from build123d import *

# Parameters (mm, degrees)
EXTRUDE_3_DEPTH = 550


with BuildPart() as part:
    # Эскиз1 → Вытянуть-Тонкостенный3 (new body)
    with BuildSketch(Plane(origin=(0, 0, 0), x_dir=(0, 0, -1), z_dir=(1, 0, 0))):
        with BuildLine():
            Line((8, 14), (8, 16))
            ThreePointArc((8, 16), (7.707106781, 16.707106781), (7, 17))
            Line((7, 17), (-0.5, 17))
            ThreePointArc((-0.5, 17), (-1.207106781, 16.707106781), (-1.5, 16))
            Line((-1.5, 16), (-1.5, 7.5))
            ThreePointArc((-1.5, 7.5), (-1.207106781, 6.792893219), (-0.5, 6.5))
            Line((-0.5, 6.5), (0, 6.5))
            Line((0, 6.5), (0, -6.5))
            Line((0, -6.5), (-0.5, -6.5))
            ThreePointArc((-0.5, -6.5), (-1.207106781, -6.792893219), (-1.5, -7.5))
            Line((-1.5, -7.5), (-1.5, -16))
            ThreePointArc((-1.5, -16), (-1.207106781, -16.707106781), (-0.5, -17))
            Line((-0.5, -17), (7, -17))
            ThreePointArc((7, -17), (7.707106781, -16.707106781), (8, -16))
            Line((8, -16), (8, -14))
            Line((8, -14), (6.8, -14))
            Line((6.8, -14), (6.8, -15.8))
            Line((6.8, -15.8), (-0.3, -15.8))
            Line((-0.3, -15.8), (-0.3, -7.7))
            Line((-0.3, -7.7), (1.2, -7.7))
            Line((1.2, -7.7), (1.2, 7.7))
            Line((1.2, 7.7), (-0.3, 7.7))
            Line((-0.3, 7.7), (-0.3, 15.8))
            Line((-0.3, 15.8), (6.8, 15.8))
            Line((6.8, 15.8), (6.8, 14))
            Line((6.8, 14), (8, 14))
        make_face()
    extrude(amount=EXTRUDE_3_DEPTH)


solid = part.part
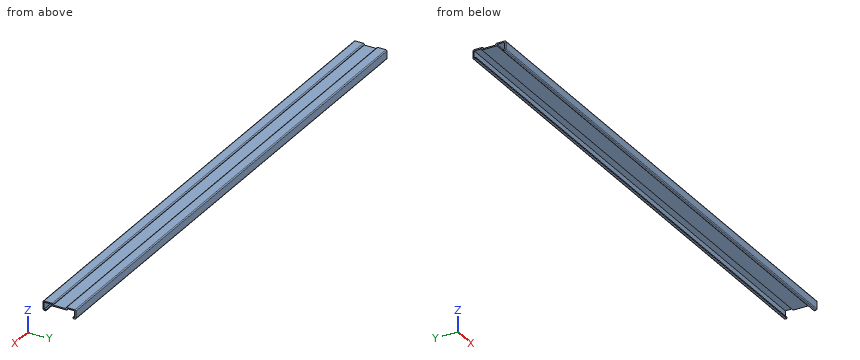
CAD build for the part. Positions are in the model's coordinates, mm. Give positions to 0.01 mm unless a question says otherwise; leave off trailing zeros. Write each loop counter-clockwise with the first axis right and the second up, starting at its lowest first coordinate (ties: lowest second). Pieces come first, ordered by that corner, then holes. Notation, with made-up numbers: (59.5, 52.5) - (101.5, 52.5) arc R33 ccw to (101.5, 83.5) - close; hole circle Ø9 at (64.5, 28.25). An arc over 180 degrees is marked (long way). Put each result on its own line as item: value.
(1) Drop flat-ended pins along their axis: pin 1 Ø6 at (x, y) = (156.5, 1.5) entering from -Z; pin 2 Ø2 at (x, y) = (332, 2) entering from +Z; pin 3 Ø4 at (x, y) = (208, -12.5) entering from -Z. Give the stop position or say it passes through.
Working result:
pin 1: z = -1.2
pin 2: z = 0
pin 3: z = -8
(2) Saw through at B-B (x = 107.5). List the corners of the cut face in (y, z).
Working result:
outline: (-17, -7) arc R1 ccw to (-16, -8) - (-14, -8) - (-14, -6.8) - (-15.8, -6.8) - (-15.8, 0.3) - (-7.7, 0.3) - (-7.7, -1.2) - (7.7, -1.2) - (7.7, 0.3) - (15.8, 0.3) - (15.8, -6.8) - (14, -6.8) - (14, -8) - (16, -8) arc R1 ccw to (17, -7) - (17, 0.5) arc R1 ccw to (16, 1.5) - (7.5, 1.5) arc R1 ccw to (6.5, 0.5) - (6.5, 0) - (-6.5, 0) - (-6.5, 0.5) arc R1 ccw to (-7.5, 1.5) - (-16, 1.5) arc R1 ccw to (-17, 0.5) - close
(3) Wall check: L1, parallel to Y at x = 65.5, z = -4.75; L2, parallel to Y at x = 397, z = 0.75; L3, parallel to Z at x = 244.5, y = 3.5. Give the ranges that are in metal, low to high.
Working result:
L1: -17 to -15.8, 15.8 to 17
L2: -16.97 to -6.53, 6.53 to 16.97
L3: -1.2 to 0
(4) Saw through at C-C (y = 1.5). List the corners of the cut face in (x, z).
Working result:
outline: (0, -1.2) - (550, -1.2) - (550, 0) - (0, 0) - close
(5) Saw through at A-A (z = -3). List the corners of the cut face in (x, y).
Working result:
outline: (0, -17) - (550, -17) - (550, -15.8) - (0, -15.8) - close; (0, 15.8) - (550, 15.8) - (550, 17) - (0, 17) - close
